from build123d import *

# Parameters (mm, degrees)
F1_DEPTH = 1.524
F2_R     = 23.0124
F2_R_2   = 1.8669
F2_R_3   = 17.2466
F2_R_4   = 1.524
F3_DEPTH = 1.525
F5_D     = 4.318


with BuildPart() as f1:
    # F0 (on Front) → F1 (new body)
    with BuildSketch(Plane.XZ):
        with BuildLine():
            Line((203.2, 0), (12.7, 0))
            ThreePointArc((12.7, 0), (3.7197438789, -3.7197438789), (0, -12.7))
            Line((0, -12.7), (0, -101.6))
            ThreePointArc((0, -101.6), (3.7197438789, -110.5802561211), (12.7, -114.3))
            Line((12.7, -114.3), (203.2, -114.3))
            ThreePointArc((203.2, -114.3), (212.1802561211, -110.5802561211), (215.9, -101.6))
            Line((215.9, -101.6), (215.9, -12.7))
            ThreePointArc((215.9, -12.7), (212.1802561211, -3.7197438789), (203.2, 0))
        make_face()
    extrude(amount=F1_DEPTH)

    # F2 (on face) → F3 (cut, through all)
    with BuildSketch(Plane.XZ.offset(1.524)):
        with Locations((53.975, -57.15)):
            Circle(F2_R)
        with Locations((34.1249, -37.2999)):
            Circle(F2_R_2)
        with Locations((73.8251, -37.2999)):
            Circle(F2_R_2)
        with Locations((73.8251, -77.0001)):
            Circle(F2_R_2)
        with Locations((34.1249, -77.0001)):
            Circle(F2_R_2)
        with Locations((161.925, -57.15)):
            Circle(F2_R_3)
        with Locations((147.2438, -42.4688)):
            Circle(F2_R_4)
        with Locations((176.6062, -42.4688)):
            Circle(F2_R_4)
        with Locations((176.6062, -71.8312)):
            Circle(F2_R_4)
        with Locations((147.2438, -71.8312)):
            Circle(F2_R_4)
        with Locations((107.95, -57.15)):
            Circle(F2_R_3)
        with Locations((93.2688, -42.4688)):
            Circle(F2_R_4)
        with Locations((122.6312, -42.4688)):
            Circle(F2_R_4)
        with Locations((122.6312, -71.8312)):
            Circle(F2_R_4)
        with Locations((93.2688, -71.8312)):
            Circle(F2_R_4)
    extrude(amount=-F3_DEPTH, mode=Mode.SUBTRACT)

    # F5 (through all)
    with Locations(Plane.XZ.offset(1.524)):
        with Locations((10.16, -9.525), (107.95, -9.525), (205.74, -9.525), (205.74, -104.775), (107.95, -104.775), (10.16, -104.775)):
            Hole(F5_D / 2)


solid = f1.part
Read the model definition and answer for the solid it produces. Units are mm, in the model's axes. Round coordinates to 2 decimals unless told otherwise and drop trailing zeros. Write each loop counter-clockwise with the first axis right and the second up, starting at its lowest first coordinate (ties: lowest second). Pieces come first, ordered by that corner, then holes. Notation, with made-up numbers: (-39, 62.25) - (-7, 62.25) arc R12 ccw to (-7, 85.25) - close; hole circle Ø9 at (22.5, -17.75). An arc over 180 degrees is marked (long way). One line per question, with ' | ' between items. Start each with the question number.
1. For a pull along Z with two mould halves and no side action, classify faces 1 (the face through (33.88, -0.77, -75.15)), 2 (the face through (130, 0, -56)), 3 (the face through (3.82, -0.75, -3.62)) as +Z half, -Z half, draft (parallel to the pull), parting line (faces both ways), or undercut.
2. Section C-C (x = 59.5) is taken. Determine the outline of the cut face in (y, z), and give its area (3 significant figures).
3. This flat-tipped pin is pushed along its axis until it touches: pin 1 (5 mm diameter, centred on x = 147.24, z = -42.47, fed in from -Y). Where does it stop, or does it pass through?
4. Section B-B (x = 107.95) is taken. Determine the outline of the cut face in (y, z), and give its area (3 significant figures).
5. Section A-A (z = -57.15) is taken. Determine the outline of the cut face in (x, y), and give its area (3 significant figures).
6. Section D-D (y = -0.65) is taken. Give the number of separate pieces and of enclosed holes in the cut face, and give its area (3 significant figures).
7. Find the intervals of material crossed by probe 1 along X at (y, z) = (-0.85, -56.5); probe 2 along X at (y, z) = (-0.65, -64.5); probe 3 along Z at (x, y) = (51.5, -0.7), in increasing order. Write a range as [from, to].
Filled in:
1) face 1: undercut | face 2: draft | face 3: +Z half
2) outline: (-1.52, -114.3) - (0, -114.3) - (0, -79.49) - (-1.52, -79.49) - close; (-1.52, -34.81) - (0, -34.81) - (0, 0) - (-1.52, 0) - close | area: 106 mm²
3) pin 1: y = -1.52
4) outline: (-1.52, -114.3) - (0, -114.3) - (0, -106.93) - (-1.52, -106.93) - close; (-1.52, -102.62) - (0, -102.62) - (0, -74.4) - (-1.52, -74.4) - close; (-1.52, -39.9) - (0, -39.9) - (0, -11.68) - (-1.52, -11.68) - close; (-1.52, -7.37) - (0, -7.37) - (0, 0) - (-1.52, 0) - close | area: 108 mm²
5) outline: (0, -1.52) - (30.96, -1.52) - (30.96, 0) - (0, 0) - close; (76.99, -1.52) - (90.7, -1.52) - (90.7, 0) - (76.99, 0) - close; (125.2, -1.52) - (144.68, -1.52) - (144.68, 0) - (125.2, 0) - close; (179.17, -1.52) - (215.9, -1.52) - (215.9, 0) - (179.17, 0) - close | area: 154 mm²
6) separate pieces: 1 | enclosed holes: 21 | area: 20,800 mm²
7) probe 1: [0, 30.97], [76.98, 90.72], [125.18, 144.69], [179.16, 215.9] | probe 2: [0, 32.17], [75.78, 92.35], [123.55, 146.32], [177.53, 215.9] | probe 3: [-114.3, -80.03], [-34.27, 0]
